```python
from build123d import *

# Parameters (mm, degrees)
F_1_BASE_W               = 100
F_1_BASE_H               = 100
RESSALTO_EXTRUS_O1_DEPTH = 15
F_2_BASE_EIXO_R          = 35
RESSALTO_EXTRUS_O2_DEPTH = 40
ESBO_O3_R                = 20
RESSALTO_EXTRUS_O3_DEPTH = 200


with BuildPart() as part:
    # 1_Base → Ressalto-extrusão1 (new body)
    with BuildSketch(Plane(origin=(0, 0, 0), x_dir=(0, 1, 0), z_dir=(0, 0, 1))):
        Rectangle(F_1_BASE_W, F_1_BASE_H)
    extrude(amount=RESSALTO_EXTRUS_O1_DEPTH)

    # 2_Base_eixo → Ressalto-extrusão2 (add)
    with BuildSketch(Plane.XY.offset(15)):
        Circle(F_2_BASE_EIXO_R)
    extrude(amount=RESSALTO_EXTRUS_O2_DEPTH)

    # Esboço3 → Ressalto-extrusão3 (add)
    with BuildSketch(Plane.XY.offset(55)):
        Circle(ESBO_O3_R)
    extrude(amount=RESSALTO_EXTRUS_O3_DEPTH)


solid = part.part
```
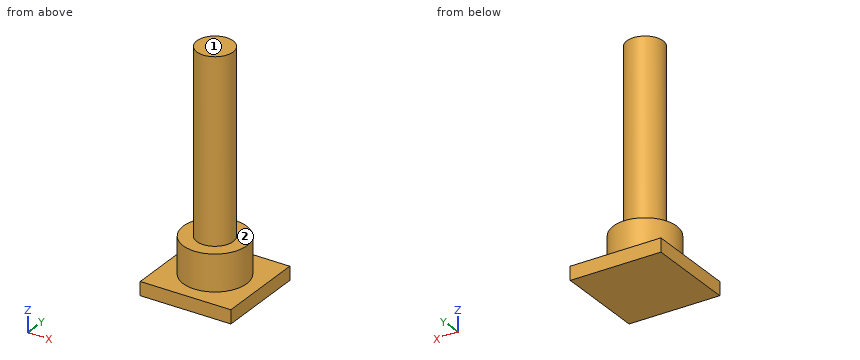
Here's how the part is built. I have some questions about the finished solid (model axes, mm). Face numbers are marked on the shaded views. A direction names the side the tool comes from. Coordinates: 2 decimals unless noted, no trailing zeros. Loops run counter-clockwise (first coordinate to the right, second up) from the corner with the lowest first, then second, coordinate; pieces in that order, holes last. Notation, with made-up numbers: (15.25, 66) - (31.25, 66) arc R24 cw to (31.25, 90) - close; hole circle Ø5 at (-6.75, 81). An arc over 180 degrees is marked (long way). Return JSON: item names as keys, results as strings. Group by question number.
Item 1: If we section it at C-C on z = 38: Write out the boundary of the cut face in (x, y), and give its area (3 significant figures).
Item 2: If we section it at A-A on x = 0: Write out the boundary of the cut face in (y, z).
Item 3: I need wall thicknesses on line 1 (Z direction, x = 38.5, y = -12); line 2 (Z direction, x = -25, y = 3); line 3 (X direction, y = -32.5, z = 32.5). Which ranges of each line are inside material? Lowest first, please. Write a range as from..to.
Item 4: Will these pins go through, and if not, where does the flat tip stop? P1, Ø6, axis at y = 13.5, z = 85.5, coming from the +X side; P2, Ø2, axis at y = 10, z = 29.5, coming from the -X side; P3, Ø10, axis at x = -16, y = 25, coming from the +Z side.
Item 5: On a 3-axis mill with a long thin cutter (end or side, diameter ignored), from which of +Z, -Z, +X, -X, +Y, -Y can I reach the whole of each face in a straight line? I mean the marked faces 1 and 2. Say none if no direction works.
Item 6: If we section it at D-D on x = -24.5: Write out the boundary of the cut face in (y, z) (3 decimals), and give its area (3 significant figures).
Calculated:
{
 "1": {"outline": "circle Ø70 at (0, 0)", "area": "3,850 mm^2"},
 "2": {"outline": "(-50, 0) - (50, 0) - (50, 15) - (35, 15) - (35, 55) - (20, 55) - (20, 255) - (-20, 255) - (-20, 55) - (-35, 55) - (-35, 15) - (-50, 15) - close"},
 "3": {"line 1": "z = 0..15", "line 2": "z = 0..55", "line 3": "x = -12.99..12.99"},
 "4": {"P1": "stops at x = 17.02", "P2": "stops at x = -33.82", "P3": "stops at z = 55"},
 "5": {"face 1": "+Z, +X, -X, +Y, -Y", "face 2": "+Z"},
 "6": {"outline": "(-50, 0) - (50, 0) - (50, 15) - (24.995, 15) - (24.995, 55) - (-24.995, 55) - (-24.995, 15) - (-50, 15) - close", "area": "3,500 mm^2"}
}
